Build history of the part. All positions in model axes, mm. Face numbers are marked on the shaded views. Round coordinates to 2 decimals unless told otherwise and drop trailing zeros. Write each loop counter-clockwise with the first axis right and the second up, starting at its lowest first coordinate (ties: lowest second). Pieces come first, ordered by that corner, then holes. Notation, with made-up numbers: (66, 39) -> (114, 39) arc R24 cw to (114, 63) -> close; hole circle Ø7 at (23.25, 54.5). An arc over 180 degrees is marked (long way). Answer as CSV lines item,"result".
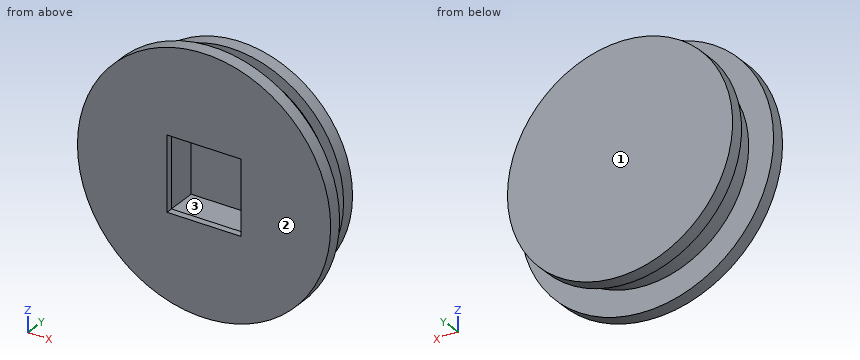
from build123d import *

# Parameters (mm, degrees)
SKETCH1_R           = 18.669
BOSS_EXTRUDE1_DEPTH = 2
SKETCH2_R           = 15
BOSS_EXTRUDE2_DEPTH = 4
SKETCH3_R           = 16.6
BOSS_EXTRUDE3_DEPTH = 2
SKETCH4_W           = 13.081
SKETCH4_H           = 13.081
CUT_EXTRUDE1_DEPTH  = 7
SKETCH5_W           = 13.081
SKETCH5_H           = 13.081
SKETCH5_W_2         = 10.922
SKETCH5_H_2         = 10.922
BOSS_EXTRUDE4_DEPTH = 1


with BuildPart() as part:
    # Sketch1 → Boss-Extrude1 (new body)
    with BuildSketch(Plane(origin=(0, 0, 0), x_dir=(1, 0, 0), z_dir=(0, 1, 0))):
        Circle(SKETCH1_R)
    extrude(amount=BOSS_EXTRUDE1_DEPTH)

    # Sketch2 → Boss-Extrude2 (add)
    with BuildSketch(Plane(origin=(0, 2, 0), x_dir=(1, 0, 0), z_dir=(0, 1, 0))):
        Circle(SKETCH2_R)
    extrude(amount=BOSS_EXTRUDE2_DEPTH)

    # Sketch3 → Boss-Extrude3 (add)
    with BuildSketch(Plane(origin=(0, 6, 0), x_dir=(1, 0, 0), z_dir=(0, 1, 0))):
        Circle(SKETCH3_R)
    extrude(amount=BOSS_EXTRUDE3_DEPTH)

    # Sketch4 → Cut-Extrude1 (cut)
    with BuildSketch(Plane(origin=(0, 0, 0), x_dir=(-1, 0, 0), z_dir=(0, -1, 0))):
        Rectangle(SKETCH4_W, SKETCH4_H)
    extrude(amount=-CUT_EXTRUDE1_DEPTH, mode=Mode.SUBTRACT)

    # Sketch5 → Boss-Extrude4 (add)
    with BuildSketch(Plane.XZ):
        Rectangle(SKETCH5_W, SKETCH5_H)
        Rectangle(SKETCH5_W_2, SKETCH5_H_2, mode=Mode.SUBTRACT)
    extrude(amount=-BOSS_EXTRUDE4_DEPTH)


solid = part.part
1. Mould opens along Y. For the marked faces 1, 2 and 3 say: +Y half, -Y half, draft (parallel to the pull), parting line (faces both ways), or undercut.
Results found:
face 1,"+Y half"
face 2,"-Y half"
face 3,"undercut"
2. Cut at D-D, the plane x = 0. Write the cut outline in (y, z), then the cut area to 3 significant figures.
Results found:
outline,"(0, -18.67) -> (2, -18.67) -> (2, -15) -> (6, -15) -> (6, -16.6) -> (8, -16.6) -> (8, 16.6) -> (6, 16.6) -> (6, 15) -> (2, 15) -> (2, 18.67) -> (0, 18.67) -> (0, 5.46) -> (1, 5.46) -> (1, 6.54) -> (7, 6.54) -> (7, -6.54) -> (1, -6.54) -> (1, -5.46) -> (0, -5.46) -> close"
area,"172 mm2"
3. Drop flat-ended pins along their axis: pin 1 Ø0.5 at (y, z) = (0.5, 2.5) entering from +X; pin 2 Ø4 at (y, z) = (1.5, -8.5) entering from -X; pin 3 Ø1.1 at (y, z) = (0.5, -2.5) entering from -X. Give the stop position or say it passes through.
Results found:
pin 1,"stops at x = 18.53"
pin 2,"stops at x = -17.5"
pin 3,"stops at x = -18.57"
4. Cut at A-A, the plane y = 4. Write the cut outline in (x, z).
Results found:
outline,"circle Ø30 at (0, 0); hole (-6.54, -6.54) -> (6.54, -6.54) -> (6.54, 6.54) -> (-6.54, 6.54) -> close"
5. Probe line 1 along Y through (x, z) = (1, 6.5); line 2 along Y through (x, z) = (-12, 11); line 3 along Y through (x, z) = (-10.5, -13.5). List the from-to ranges inside material, lowest first.
Results found:
line 1,"y = 0 to 1, 7 to 8"
line 2,"y = 0 to 2, 6 to 8"
line 3,"y = 0 to 2"
6. Cut at B-B, the plane x = 16. Write the cut outline in (y, z), then the cut area to 3 significant figures.
Results found:
outline,"(0, -9.62) -> (2, -9.62) -> (2, 9.62) -> (0, 9.62) -> close; (6, -4.42) -> (8, -4.42) -> (8, 4.42) -> (6, 4.42) -> close"
area,"56.2 mm2"
7. Cut at C-C, the plane z = 0. Write the cut outline in (x, y).
Results found:
outline,"(-18.67, 0) -> (-5.46, 0) -> (-5.46, 1) -> (-6.54, 1) -> (-6.54, 7) -> (6.54, 7) -> (6.54, 1) -> (5.46, 1) -> (5.46, 0) -> (18.67, 0) -> (18.67, 2) -> (15, 2) -> (15, 6) -> (16.6, 6) -> (16.6, 8) -> (-16.6, 8) -> (-16.6, 6) -> (-15, 6) -> (-15, 2) -> (-18.67, 2) -> close"
